Build history of the part. All positions in model axes, mm. Give positions to 0.01 mm unless a question says otherwise; leave off trailing zeros. Loops run counter-clockwise (first coordinate to the right, second up) from the corner with the lowest first, then second, coordinate; pieces in that order, holes last.
1) Wall check: line 1 (Y direction, x = -8, z = 3.5); line 2 (Y direction, x = 10, z = 7.25); line 3 (Y direction, x = -15.5, z = 3). Give the ranges that are in metal, low to high.
2) Band-saw the part on A-A on z = 5. State how many separate pieces and enclosed holes the cut face has, then the cut area to 3 significant figures.
3) Flat gauge pins, fed straight in: P1, Ø4, axis at y = 2, z = 10, coming from the +X side (3 decimals); P2, Ø1.4, axis at x = 15.875, y = 0, coming from the -Z side; P3, Ø2.5, axis at x = 23.81, y = 0, coming from the +Z side (3 decimals); P4, Ø1.3, axis at x = -43.66, y = 0, coming from the -Z side (3 decimals). Where does each tip first touch, or does it go through?
4) Band-saw the part on B-B on x = 31.75. List the corners of the cut face in (y, z) (1 decimal).
```python
from build123d import *

# Parameters (mm, degrees)
F0_W     = 95.25
F0_H     = 7.9375
F0_R     = 2.38125
F1_DEPTH = 9.525
F2_DEPTH = 11.1125
F3_T     = -1.5875
F4_R     = 1.5875
F4_R_2   = 0.79375
F5_DEPTH = 7.9375


# Not quite as in the source:
# - a feature names something its author has since deleted; it is built from what else it names


with BuildPart() as f1:
    # F0 (on Top) → F1 (new body)
    with BuildSketch(Plane.XY):
        Rectangle(F0_W, F0_H)
        with Locations((-43.65625, 0)):
            Circle(F0_R, mode=Mode.SUBTRACT)
        with Locations((-35.71875, 0)):
            Circle(F0_R, mode=Mode.SUBTRACT)
        with Locations((-27.78125, 0)):
            Circle(F0_R, mode=Mode.SUBTRACT)
        with Locations((-19.84375, 0)):
            Circle(F0_R, mode=Mode.SUBTRACT)
        with Locations((-11.90625, 0)):
            Circle(F0_R, mode=Mode.SUBTRACT)
        with Locations((-3.96875, 0)):
            Circle(F0_R, mode=Mode.SUBTRACT)
        with Locations((3.96875, 0)):
            Circle(F0_R, mode=Mode.SUBTRACT)
        with Locations((11.90625, 0)):
            Circle(F0_R, mode=Mode.SUBTRACT)
        with Locations((19.84375, 0)):
            Circle(F0_R, mode=Mode.SUBTRACT)
        with Locations((27.78125, 0)):
            Circle(F0_R, mode=Mode.SUBTRACT)
        with Locations((35.71875, 0)):
            Circle(F0_R, mode=Mode.SUBTRACT)
        with Locations((43.65625, 0)):
            Circle(F0_R, mode=Mode.SUBTRACT)
    extrude(amount=F1_DEPTH)

    # F0 (on Top) → F2 (join)
    with BuildSketch(Plane.XY):
        with Locations((-43.65625, 0)):
            Circle(F0_R)
        with Locations((-35.71875, 0)):
            Circle(F0_R)
        with Locations((-27.78125, 0)):
            Circle(F0_R)
        with Locations((-19.84375, 0)):
            Circle(F0_R)
        with Locations((-11.90625, 0)):
            Circle(F0_R)
        with Locations((-3.96875, 0)):
            Circle(F0_R)
        with Locations((3.96875, 0)):
            Circle(F0_R)
        with Locations((11.90625, 0)):
            Circle(F0_R)
        with Locations((19.84375, 0)):
            Circle(F0_R)
        with Locations((27.78125, 0)):
            Circle(F0_R)
        with Locations((35.71875, 0)):
            Circle(F0_R)
        with Locations((43.65625, 0)):
            Circle(F0_R)
    extrude(amount=F2_DEPTH)

    # F3
    f3_openings = [f1.faces().sort_by_distance(p)[0] for p in [
        (0, 0, 0),
    ]]
    offset(amount=F3_T, openings=f3_openings, kind=Kind.INTERSECTION)

    # F4 (on face) → F5 (join)
    with BuildSketch(Plane(origin=(0, 0, 7.9375), x_dir=(1, 0, 0), z_dir=(0, 0, -1))):
        with Locations((-39.6875, 0)):
            Circle(F4_R)
        with Locations((-39.6875, 0)):
            Circle(F4_R_2, mode=Mode.SUBTRACT)
        with Locations((-31.75, 0)):
            Circle(F4_R)
        with Locations((-31.75, 0)):
            Circle(F4_R_2, mode=Mode.SUBTRACT)
        with Locations((-23.8125, 0)):
            Circle(F4_R)
        with Locations((-23.8125, 0)):
            Circle(F4_R_2, mode=Mode.SUBTRACT)
        with Locations((-15.875, 0)):
            Circle(F4_R)
        with Locations((-15.875, 0)):
            Circle(F4_R_2, mode=Mode.SUBTRACT)
        with Locations((-7.9375, 0)):
            Circle(F4_R)
        with Locations((-7.9375, 0)):
            Circle(F4_R_2, mode=Mode.SUBTRACT)
        Circle(F4_R)
        Circle(F4_R_2, mode=Mode.SUBTRACT)
        with Locations((7.9375, 0)):
            Circle(F4_R)
        with Locations((7.9375, 0)):
            Circle(F4_R_2, mode=Mode.SUBTRACT)
        with Locations((15.875, 0)):
            Circle(F4_R)
        with Locations((15.875, 0)):
            Circle(F4_R_2, mode=Mode.SUBTRACT)
        with Locations((23.8125, 0)):
            Circle(F4_R)
        with Locations((23.8125, 0)):
            Circle(F4_R_2, mode=Mode.SUBTRACT)
        with Locations((31.75, 0)):
            Circle(F4_R)
        with Locations((31.75, 0)):
            Circle(F4_R_2, mode=Mode.SUBTRACT)
        with Locations((39.6875, 0)):
            Circle(F4_R)
        with Locations((39.6875, 0)):
            Circle(F4_R_2, mode=Mode.SUBTRACT)
    extrude(amount=F5_DEPTH)


solid = f1.part
```
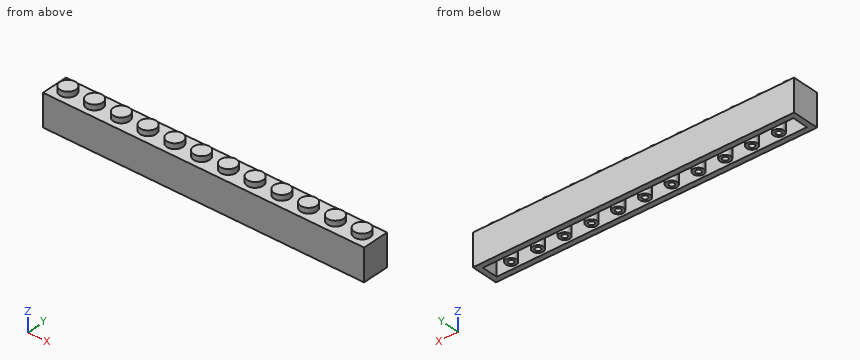
Findings below:
1. line 1: y = -3.97 to -2.38, -1.59 to -0.79, 0.79 to 1.59, 2.38 to 3.97
1. line 2: y = -3.97 to -2.38, 2.38 to 3.97
1. line 3: y = -3.97 to -2.38, -1.54 to -0.7, 0.7 to 1.54, 2.38 to 3.97
2. separate pieces: 12
2. enclosed holes: 12
2. area: 383 mm2
3. P1: stops at x = 47.625
3. P2: stops at z = 7.94
3. P3: stops at z = 9.525
3. P4: stops at z = 9.525
4. outline: (-4, 0) - (-2.4, 0) - (-2.4, 7.9) - (-1.6, 7.9) - (-1.6, 0) - (-0.8, 0) - (-0.8, 7.9) - (0.8, 7.9) - (0.8, 0) - (1.6, 0) - (1.6, 7.9) - (2.4, 7.9) - (2.4, 0) - (4, 0) - (4, 9.5) - (-4, 9.5) - close
